Geometry: final body of the model. Coordinates: model frame, mm. A direction names the side the tool comes from. Coordinates: 2 decimals unless noted, no trailing zeros. Order: outer loops, then holes, each group sorted by start corner. A loop starts at its lowest first (then second) coordinate and runs counter-clockwise, first axis right, second up. Notation, with made-up numbers: (87, 88) -> (111, 88) arc R21 ccw to (111, 122) -> close; hole circle Ø9 at (78.5, -20.5). An arc over 180 degrees is marked (long way). Use one line per item in the form item = value.
Autodesk Inventor part; units mm, degrees
ref_plane "Work Plane1" through (30, 0, 0) normal (0, -0.5, 0.866) x (1, 0, 0)
ref_plane "YZ Plane" through (0, 0, 0) normal (1, 0, 0) x (0, 1, 0)
ref_plane "XZ Plane" through (0, 0, 0) normal (0, 1, 0) x (-1, 0, 0)
sketch "Sketch1" plane through (0, 0, 0) normal (0, 0, 1) x (1, 0, 0)
  line L0 (0.1133, 0) -> (10, 0)
  line L1 (10, 0) -> (10, 3)
  line L2 (10, 3) -> (2, 3)
  line L3 (2, 3) -> (1.3865, 3)
  line L4 (1.3865, 3) -> (0, 3)
  line L5 (0, 3) -> (0, 5.25)
  line L6 (0, 5.25) -> (-3.3, 5.25)
  line L7 (-3.3, 5.25) -> (-3.3, 2.3094)
  line L8 (-3.3, 2.3094) -> (-1.22, 2.3094)
  line L9 (-1.22, 2.3094) -> (0.1133, 0)
  line L10 (-5.96, 0) -> (12.66, 0)
  line L11 (0, -1.05) -> (0, 6.3)
  line L12 (2, 3) -> (0, 3) construction
  dimension "d0" = 8
  dimension "d1" = 0.6135
  dimension "d2" = 3.3
  dimension "d3" = 2.08
  dimension "d4" = 60
  dimension "d5" = 6
  dimension "d6" = 6
  dimension "d7" = 4.6188
  dimension "d8" = 10.5
  dimension "d19" = 10
revolve "Body" add sketch "Sketch1" angle 360 about axis through (0.1133, 0, 0) along (1, 0, 0) contours L9 L11 L4 L3 L2 L1 L0 | L9 L8 L7 L6 L5 L11
sketch "Sketch2" plane through (-3.3, 0, 0) normal (-1, 0, 0) x (0, 0, 1)
  circle A0 centre (0, 0) radius 2.3094
  line L0 (0, -7.35) -> (0, 7.35)
  line L1 (-7.35, 0) -> (7.35, 0)
  line L2 (2.3094, 0) -> (1.1547, -2)
  line L3 (1.1547, -2) -> (-1.1547, -2)
  line L4 (-1.1547, -2) -> (-2.3094, 0)
  line L5 (-2.3094, 0) -> (-1.1547, 2)
  line L6 (-1.1547, 2) -> (1.1547, 2)
  line L7 (1.1547, 2) -> (2.3094, 0)
extrude "Slot" add sketch "Sketch2" against normal up to next contours L7 A0 | A0 L2 | L6 L0 A0 | A0 L0 L3 | L0 L6 A0 | A0 L3 L0 | L4 A0 | A0 L5
fillet "Fillet1" radius 2.625 1 edges at (-3.3, -5.25, 0)
thread "Thread"
chamfer "Chamfer1" distance 0.6135 distance2 0.6135 1 edges at (10, -3, 0) measured on face at (10, 0.705, 0.3049)
fillet "Fillet2" radius 0.25 1 edges at (0, -3, 0)
ref_plane "Work Plane1" through (30, 0, 0) normal (0, -0.5, 0.866) x (1, 0, 0)
equation "\"d0\" = GEL"
equation "\"d1\" = GAL"
equation "\"d2\" = KOH"
equation "\"d3\" = INTI"
equation "\"d5\" = GD"
equation "\"d6\" = BDM"
equation "\"d7\" = 1.1547 * SW"
equation "\"d8\" = KOD"
equation "\"d19\" = NLG"
equation "\"d16\" = RR"
equation "\"d12\" = GEL"
equation "\"d14\" = -0.5 * SPD + 0.5 * GD"
equation "\"d15\" = GUL"
equation "\"d29\" = R"
equation "\"GD\" = NND"
equation "\"NLG\" = 10"
equation "\"GEL\" = 8"
equation "\"KOD\" = 10.5"
equation "\"KOH\" = 3.3"
equation "\"INTI\" = 2.08"
equation "\"GAL\" = 0.61345 * PTC"
equation "\"GUL\" = 0.61345 * PTC"
equation "\"BDM\" = NND"
equation "\"SW\" = 4"
equation "\"RR\" = 2.625"
equation "\"SPD\" = 4.7731"
equation "\"d28\" = R"
equation "\"R\" = 0.25"
equation "\"TOA\" = 30deg"
equation "\"THREADDIA\" = 6"
equation "\"KOD1\" = KOD - 2 * RR"
equation "\"PTC\" = 1"
equation "\"NND\" = 6"
equation "\"E0\" = 1.155 * SW"
equation "\"GD1\" = THREADDIA - 1.2269 * PTC"
properties part number "ANSI B18.3.4M - M6 x 1 x 10" material "Steel, Mild"
1) Pull-direction query (Y, two-part tool) for faces 3 (the cylindrical face through (5, -3, 0)), 4 (the flat face through (-2, 2, 0)), 5 (the conical face through (0.03, 0.14, -0.04)), 6 (the flat face through (0, -0.1, -3.4)); classes: released by +Y, released by -Y, zero draft, split by the parting line, or undercut.
Results found:
face_3 = split by the parting line
face_4 = undercut
face_5 = undercut
face_6 = zero draft
2) Material intervals for probe 1 along Z at (x, y) = (-2.5, -0.25); probe 2 along Z at (x, y) = (-1.5, 1.5); probe 3 along X at (y, z) = (3.75, 1.75), sorted ascending. Write a range as from..to.
Results found:
probe_1 = -4.5..-2.17, 2.17..4.5
probe_2 = -4.89..-1.44, 1.44..4.89
probe_3 = -2.82..0
3) Section A-A, the plane x = 1.5. Output: boundary loops of the cut face in (y, z), and give its area (3 significant figures).
Results found:
outline = circle Ø6 at (0, 0)
area = 28.3 mm2
4) Contact query for flat-ended pins moving along their axis: P1, Ø2.5, axis at x = -2, z = -0.5, coming from the -Y side; P2, Ø5, axis at y = 4, z = 3.5, coming from the -X side; P3, Ø2.5, axis at x = -2, z = 0.5, coming from the +Y side; P4, Ø5, axis at y = 3.5, z = 3, coming from the +X side. Output: stop coordinate, or through.
Results found:
P1 = -5.25
P2 = -3.29
P3 = 5.25
P4 = 10
5) Access query for faces 1 (the flat face through (10, 0, 0)), 2 (the flat face through (-2, -2, 0)). Directions: +Z, -Z, +X, -X, +Y, -Y. A direction counts if a zero-diameter tool reaches every point of the face in a straight line with its end or side. Return the directions, or none.
Results found:
face_1 = +Z, -Z, +X, +Y, -Y
face_2 = -X
